Here's how the part is built. I have some questions about the finished solid (model axes, mm). Coordinates: 2 decimals unless noted, no trailing zeros. Write each loop counter-clockwise with the first axis right and the second up, starting at its lowest first coordinate (ties: lowest second). Pieces come first, ordered by that corner, then holes. Notation, with made-up numbers: M 59.5,68.5 L 84.5,68.5 A28 cw 84.5,87.5 Z; hole C 44.5,84 d8. An arc over 180 degrees is marked long. Use a Markdown table: item, result.
```python
from build123d import *

# Parameters (mm, degrees)
SKETCH2_W           = 139
SKETCH2_H           = 90
SKETCH2_W_2         = 60
SKETCH2_H_2         = 80
BOSS_EXTRUDE1_DEPTH = 5
CUT_EXTRUDE5_DEPTH  = 5
CUT_EXTRUDE6_START  = 134
CUT_EXTRUDE6_DEPTH  = 5
SKETCH12_W          = 2.75
SKETCH12_H          = 19
BOSS_EXTRUDE2_DEPTH = 5


with BuildPart() as part:
    # Sketch2 → Boss-Extrude1 (new body)
    with BuildSketch(Plane(origin=(0, 0, 0), x_dir=(0, 1, 0), z_dir=(0, 0, 1))):
        Rectangle(SKETCH2_W, SKETCH2_H)
        with Locations((33.5, 0)):
            Rectangle(SKETCH2_W_2, SKETCH2_H_2, mode=Mode.SUBTRACT)
        with Locations((-33.5, 0)):
            Rectangle(SKETCH2_W_2, SKETCH2_H_2, mode=Mode.SUBTRACT)
    extrude(amount=BOSS_EXTRUDE1_DEPTH)

    # Sketch13 → Cut-Extrude5 (cut)
    with BuildSketch(Plane(origin=(0, -69.5, -60), x_dir=(1, 0, 0), z_dir=(0, 1, 0))):
        Polygon((-13.423393759, -60), (13.423393759, -60), (0, -83.25), align=None)
    extrude(amount=CUT_EXTRUDE5_DEPTH, mode=Mode.SUBTRACT)

    # Sketch13<3> → Cut-Extrude6 (cut)
    with BuildSketch(Plane(origin=(0, -69.5, -60), x_dir=(1, 0, 0), z_dir=(0, 1, 0)).offset(CUT_EXTRUDE6_START)):
        Polygon((-13.423393759, -60), (13.423393759, -60), (0, -83.25), align=None)
    extrude(amount=CUT_EXTRUDE6_DEPTH, mode=Mode.SUBTRACT)

    # Sketch12 → Boss-Extrude2 (add)
    with BuildSketch(Plane.XY.offset(5)):
        Polygon((-50, 32.519237886), (-45, 35.405989232), (-45, 55.613248654), (-50, 58.5), align=None)
        Polygon((-45, -10.103629711), (-45, 10.103629711), (-50, 12.990381057), (-50, -12.990381057), align=None)
        with Locations((-38.625, 33.5)):
            Rectangle(SKETCH12_W, SKETCH12_H)
        Polygon((-45, -55.613248654), (-45, -35.405989232), (-50, -32.519237886), (-50, -58.5), align=None)
        Polygon((-16.454482672, 6.25), (-14.866769432, 3.5), (14.866769432, 3.5), (16.454482672, 6.25), align=None)
        with Locations((-38.625, -33.5)):
            Rectangle(SKETCH12_W, SKETCH12_H)
        Polygon((14.866769432, 63.5), (-14.866769432, 63.5), (-16.454482672, 60.75), (16.454482672, 60.75), align=None)
        Polygon((-14.866769432, -3.5), (-16.454482672, -6.25), (16.454482672, -6.25), (14.866769432, -3.5), align=None)
        Polygon((-16.454482672, -60.75), (-14.866769432, -63.5), (14.866769432, -63.5), (16.454482672, -60.75), align=None)
        Polygon((50, 58.5), (45, 55.613248654), (45, 35.405989232), (50, 32.519237886), align=None)
        with Locations((38.625, 33.5)):
            Rectangle(SKETCH12_W, SKETCH12_H)
        Polygon((45, -35.405989232), (45, -55.613248654), (50, -58.5), (50, -32.519237886), align=None)
        with Locations((38.625, -33.5)):
            Rectangle(SKETCH12_W, SKETCH12_H)
        Polygon((45, 10.103629711), (45, -10.103629711), (50, -12.990381057), (50, 12.990381057), align=None)
    extrude(amount=-BOSS_EXTRUDE2_DEPTH)


solid = part.part
```
1. We'd pull the mould along Y, two halves only. Please class faces 1 (the face through (-50, 46, 3)), 2 (the face through (-28, -69.5, 2)), 3 (the face through (39, 43, 3)): +Y half, -Y half, draft (parallel to the pull), parting line (faces both ways), or undercut.
Answers follow:
| item | result |
|---|---|
| face 1 | draft |
| face 2 | -Y half |
| face 3 | undercut |
2. Will this pin go through, and if not, where does the flat tip stop? pin 1 Ø1.5 at (y, z) = (-61.5, 3) entering from +X.
Answers follow:
| item | result |
|---|---|
| pin 1 | stops at x = 45 |
3. Suppose I cut it at D-D on z = 0.75. State how many separate pieces and enclosed holes the cut face has, and give its area (3 significant figures).
Answers follow:
| item | result |
|---|---|
| separate pieces | 1 |
| enclosed holes | 2 |
| area | 3,900 mm2 |
4. I need wall thicknesses on probe 1 along Y at (x, z) = (21.5, 2.85); probe 2 along Y at (x, z) = (-1, 4.25); probe 3 along X at (y, z) = (50.5, 1.6). Which ranges of each line are inside material? Lowest first, please.
Answers follow:
| item | result |
|---|---|
| probe 1 | y = -69.5 to -63.5, -3.5 to 3.5, 63.5 to 69.5 |
| probe 2 | y = -64.5 to -60.75, -6.25 to 6.25, 60.75 to 64.5 |
| probe 3 | x = -50 to -40, 40 to 50 |
5. Suppose I cut it at A-A on y = -27.5. Write out the boundary of the cut face in (x, z).
Answers follow:
| item | result |
|---|---|
| outline | M -45,0 L -37.25,0 L -37.25,5 L -45,5 Z; M 37.25,0 L 45,0 L 45,5 L 37.25,5 Z |
6. Suppose I cut it at C-C on x = 5. Write out the boundary of the cut face in (y, z), and give its area (3 significant figures).
Answers follow:
| item | result |
|---|---|
| outline | M -64.5,0 L -60.75,0 L -60.75,5 L -64.5,5 Z; M -6.25,0 L 6.25,0 L 6.25,5 L -6.25,5 Z; M 60.75,0 L 64.5,0 L 64.5,5 L 60.75,5 Z |
| area | 100 mm2 |
7. Suppose I cut it at B-B on x = -20.5. Write out the boundary of the cut face in (y, z).
Answers follow:
| item | result |
|---|---|
| outline | M -69.5,0 L -63.5,0 L -63.5,5 L -69.5,5 Z; M -3.5,0 L 3.5,0 L 3.5,5 L -3.5,5 Z; M 63.5,0 L 69.5,0 L 69.5,5 L 63.5,5 Z |
